from build123d import *

# Parameters (mm, degrees)
SKETCH_1_W                = 10
SKETCH_1_H                = 14
EXTRUDE_1_DEPTH           = 37
EXTRUDE_3_DEPTH           = 7
SKETCH_8_W                = 12.090263245
SKETCH_8_H                = 10.07196207
CUT_EXTRUDE_3_DEPTH       = 5
SKETCH_10_R               = 2.5
CUT_EXTRUDE_4_DEPTH       = 8
CUT_EXTRUDE_4_DEPTH_BACK  = 8
SKETCH_14_W               = 10
SKETCH_14_H               = 10
CUT_EXTRUDE_8_DEPTH       = 3
SKETCH_15_W               = 10
SKETCH_15_H               = 10
EXTRUDE_4_DEPTH           = 3
SKETCH_16_R               = 2.5
CUT_EXTRUDE_9_DEPTH       = 8
CUT_EXTRUDE_9_DEPTH_BACK  = 8
SKETCH_17_R               = 2.5
CUT_EXTRUDE_10_DEPTH      = 8
CUT_EXTRUDE_10_DEPTH_BACK = 8


with BuildPart() as part:
    # 草图1 → 凸台-拉伸1 (new body, symmetric)
    with BuildSketch(Plane(origin=(0, 0, 0), x_dir=(1, 0, 0), z_dir=(0, 1, 0))):
        Rectangle(SKETCH_1_W, SKETCH_1_H)
    extrude(amount=EXTRUDE_1_DEPTH, both=True)

    # 草图7 → 凸台-拉伸3 (add, symmetric)
    with BuildSketch(Plane.XY):
        Polygon((5, 5), (17, 5), (17.090263245, -5.07196207), (5, -5.07196207), align=None)
    extrude(amount=EXTRUDE_3_DEPTH, both=True)

    # 草图8 → 切除-拉伸3 (cut, symmetric)
    with BuildSketch(Plane.XY):
        with Locations((11.045131623, -0.035981035)):
            Rectangle(SKETCH_8_W, SKETCH_8_H)
    extrude(amount=CUT_EXTRUDE_3_DEPTH, both=True, mode=Mode.SUBTRACT)

    # 草图10 → 切除-拉伸4 (cut, two sides)
    with BuildSketch(Plane.XY) as cut_extrude_4_sk:
        with Locations((12, 0)):
            Circle(SKETCH_10_R)
    extrude(amount=CUT_EXTRUDE_4_DEPTH, mode=Mode.SUBTRACT)
    extrude(cut_extrude_4_sk.sketch, amount=-CUT_EXTRUDE_4_DEPTH_BACK, mode=Mode.SUBTRACT)

    # 草图14 → 切除-拉伸8 (cut, symmetric)
    with BuildSketch(Plane.XY):
        with Locations((0, 32)):
            Rectangle(SKETCH_14_W, SKETCH_14_H)
    extrude(amount=CUT_EXTRUDE_8_DEPTH, both=True, mode=Mode.SUBTRACT)

    # 草图15 → 凸台-拉伸4 (add, symmetric)
    with BuildSketch(Plane.XY):
        with Locations((0, -42)):
            Rectangle(SKETCH_15_W, SKETCH_15_H)
    extrude(amount=EXTRUDE_4_DEPTH, both=True)

    # 草图16 → 切除-拉伸9 (cut, two sides)
    with BuildSketch(Plane.XY) as cut_extrude_9_sk:
        with Locations((0, 33)):
            Circle(SKETCH_16_R)
    extrude(amount=CUT_EXTRUDE_9_DEPTH, mode=Mode.SUBTRACT)
    extrude(cut_extrude_9_sk.sketch, amount=-CUT_EXTRUDE_9_DEPTH_BACK, mode=Mode.SUBTRACT)

    # 草图17 → 切除-拉伸10 (cut, two sides)
    with BuildSketch(Plane.XY) as cut_extrude_10_sk:
        with Locations((0, -43)):
            Circle(SKETCH_17_R)
    extrude(amount=CUT_EXTRUDE_10_DEPTH, mode=Mode.SUBTRACT)
    extrude(cut_extrude_10_sk.sketch, amount=-CUT_EXTRUDE_10_DEPTH_BACK, mode=Mode.SUBTRACT)


solid = part.part
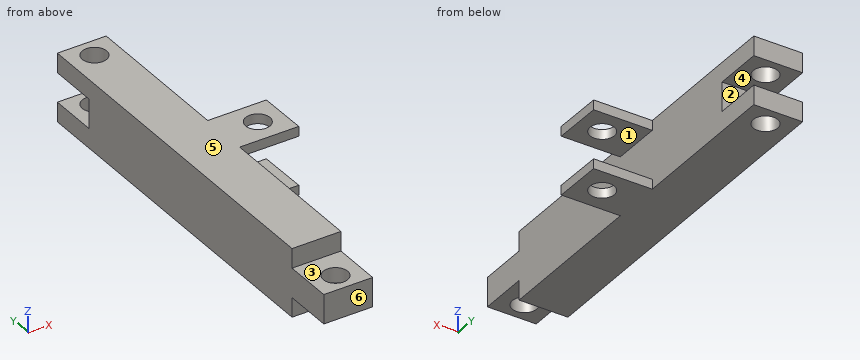
Geometry check sheet. Reference: the model listing, model coordinates, mm. Face numbers are marked on the shaded views. A direction names the side the tool comes from. Give positions to 0.01 mm unless a question says otherwise; leave off trailing zeros. Write each loop counter-clockwise with the first axis right and the second up, starting at its lowest first coordinate (ties: lowest second). Pieces come first, ordered by that corner, then holes.
1) Cross-section at B-B (y = -43). Record the boundary of the cut face in (x, z), plus the area to 3 significant figures.
Values follow:
outline: (-5, -3) - (-2.5, -3) - (-2.5, 3) - (-5, 3) - close; (2.5, -3) - (5, -3) - (5, 3) - (2.5, 3) - close
area: 30.0 mm2
2) Cross-section at D-D (x = 12). Record the boundary of the cut face in (y, z).
Values follow:
outline: (-5.07, -7) - (-2.5, -7) - (-2.5, -5) - (-5.07, -5) - close; (-5.07, 5) - (-2.5, 5) - (-2.5, 7) - (-5.07, 7) - close; (2.5, -7) - (5, -7) - (5, -5) - (2.5, -5) - close; (2.5, 5) - (5, 5) - (5, 7) - (2.5, 7) - close
3) Cross-section at A-A (x = 0). Record the boundary of the cut face in (y, z).
Values follow:
outline: (-47, -3) - (-45.5, -3) - (-45.5, 3) - (-47, 3) - close; (-40.5, -3) - (-37, -3) - (-37, -7) - (30.5, -7) - (30.5, -3) - (27, -3) - (27, 3) - (30.5, 3) - (30.5, 7) - (-37, 7) - (-37, 3) - (-40.5, 3) - close; (35.5, -7) - (37, -7) - (37, -3) - (35.5, -3) - close; (35.5, 3) - (37, 3) - (37, 7) - (35.5, 7) - close
4) Set-up check for the marked faces 1, 2 and 3: record each of +Z, -Z, +X, -X, +Y, -Y from which the full face is reachable in a straight line by a thin tool's end or side.
Values follow:
face 1: +X, +Y, -Y
face 2: +X, -X, +Y
face 3: +Z, +X, -X, -Y
5) Thickness scan on line 1 (Z direction, x = 6.25, y = 0); line 2 (Y direction, x = 12, z = 5.6); line 3 (Y direction, x = 0, z = -0.25). Record the ranges inside material, lowest first.
Values follow:
line 1: z = -7 to -5, 5 to 7
line 2: y = -5.07 to -2.5, 2.5 to 5
line 3: y = -47 to -45.5, -40.5 to 27
6) Cross-section at C-C (z = -3.75). Record the boundary of the cut face in (x, y), plus the area to 3 significant figures.
Values follow:
outline: (-5, -37) - (5, -37) - (5, 37) - (-5, 37) - close; hole circle Ø5 at (0, 33)
area: 720 mm2
7) Go/stop test with flat-tipped pins: pin 1 Ø2 at (x, z) = (10, 6) entering from +Y; pin 2 Ø1.6 at (x, z) = (11, 6) entering from -Y; pin 3 Ø1 at (y, z) = (21.5, -3) entering from +X. Record where each tip stops, or that it passes through.
Values follow:
pin 1: stops at y = 5
pin 2: stops at y = -5.07
pin 3: stops at x = 5
8) Release check for a two-part mould opening along Z. For the marked faces 4, 5 and 6 record: released by +Z, released by -Z, zero draft, split by the parting line, or undercut.
Values follow:
face 4: undercut
face 5: released by +Z
face 6: zero draft
